```python
from build123d import *

# Parameters (mm, degrees)
SKETCH1_W           = 38.1
SKETCH1_H           = 88.9
BOSS_EXTRUDE1_DEPTH = 584.2
SKETCH2_R           = 12.7
CUT_EXTRUDE1_DEPTH  = 593.152395925
SKETCH2_3_W         = 88.9
SKETCH2_3_H         = 584.2
SKETCH2_3_R         = 12.7
CUT_EXTRUDE2_DEPTH  = 3.175


with BuildPart() as part:
    # Sketch1 → Boss-Extrude1 (new body)
    with BuildSketch(Plane(origin=(0, 0, 0), x_dir=(1, 0, 0), z_dir=(0, 1, 0))):
        with Locations((19.05, 44.45)):
            Rectangle(SKETCH1_W, SKETCH1_H)
    extrude(amount=BOSS_EXTRUDE1_DEPTH)

    # Sketch2 → Cut-Extrude1 (cut, through all)
    with BuildSketch(Plane(origin=(38.1, 0, 0), x_dir=(0, 0, -1), z_dir=(1, 0, 0))):
        with Locations((37.01034, 76.2)):
            Circle(SKETCH2_R)
        with Locations((37.01034, 508)):
            Circle(SKETCH2_R)
    extrude(amount=-CUT_EXTRUDE1_DEPTH, mode=Mode.SUBTRACT)

    # Sketch2<3> → Cut-Extrude2 (cut)
    with BuildSketch(Plane(origin=(38.1, 0, 0), x_dir=(0, 0, -1), z_dir=(1, 0, 0))):
        with Locations((44.45, 292.1)):
            Rectangle(SKETCH2_3_W, SKETCH2_3_H)
        with Locations((37.01034, 76.2)):
            Circle(SKETCH2_3_R, mode=Mode.SUBTRACT)
        with Locations((37.01034, 508)):
            Circle(SKETCH2_3_R, mode=Mode.SUBTRACT)
    extrude(amount=-CUT_EXTRUDE2_DEPTH, mode=Mode.SUBTRACT)


solid = part.part
```
Read the model definition and answer for the solid it produces. Units are mm, in the model's axes. Give positions to 0.01 mm unless a question says otherwise; leave off trailing zeros. Write each loop counter-clockwise with the first axis right and the second up, starting at its lowest first coordinate (ties: lowest second). Pieces come first, ordered by that corner, then holes. Notation, with made-up numbers: (27.5, 41.25) - (47.5, 41.25) arc R11 cw to (47.5, 49.25) - close; hole circle Ø7 at (45, 66.5). An arc over 180 degrees is marked (long way). Write item = value, one per line. Start each with the question number.
Item 1: Find section B-B (z = -39). Give the vertices of the cut face in (x, y) (3 decimals).
Item 2: Find section D-D (y = 515.5). Give the vertices of the cut face in (x, z) (3 decimals).
Item 3: Find section C-C (x = 29.5). Give the vertices of the cut face in (y, z), then the cut area to 3 significant figures.
Item 4: Find section A-A (y = 76.2). Give the vertices of the cut face in (x, z) (3 decimals), then the cut area to 3 significant figures.
Item 5: Find the intervals of material crossed by probe 1 along Y at (x, z) = (5, -38.5); probe 2 along Y at (x, z) = (3.5, -34.5), in increasing order. Write a range as [from, to].
Item 6: The mould has two halves that part along Y. Classify faces 1 (the flat face through (17, 288, -88.9)), 2 (the cylindrical face through (17.71, 63.8, -34.26)), 3 (the flat face through (17, 584.2, -45)), 4 (the flat face through (17, 0, -45)): +Y half, -Y half, draft (parallel to the pull), parting line (faces both ways), or undercut.
Response:
q1.outline = (0, 0) - (34.925, 0) - (34.925, 63.657) - (0, 63.657) - close; (0, 88.743) - (34.925, 88.743) - (34.925, 495.457) - (0, 495.457) - close; (0, 520.543) - (34.925, 520.543) - (34.925, 584.2) - (0, 584.2) - close
q2.outline = (0, -88.9) - (34.925, -88.9) - (34.925, -47.259) - (0, -47.259) - close; (0, -26.761) - (34.925, -26.761) - (34.925, 0) - (0, 0) - close
q3.outline = (0, -88.9) - (584.2, -88.9) - (584.2, 0) - (0, 0) - close; hole circle Ø25.4 at (76.2, -37.01); hole circle Ø25.4 at (508, -37.01)
q3.area = 50,900 mm²
q4.outline = (0, -88.9) - (34.925, -88.9) - (34.925, -49.71) - (0, -49.71) - close; (0, -24.31) - (34.925, -24.31) - (34.925, 0) - (0, 0) - close
q4.area = 2,220 mm²
q5.probe_1 = [0, 63.59], [88.81, 495.39], [520.61, 584.2]
q5.probe_2 = [0, 63.75], [88.65, 495.55], [520.45, 584.2]
q6.face_1 = draft
q6.face_2 = undercut
q6.face_3 = +Y half
q6.face_4 = -Y half
